Autodesk Inventor part; units mm, degrees
ref_plane "YZ Plane" through (0, 0, 0) normal (1, 0, 0) x (0, 1, 0)
ref_plane "XZ Plane" through (0, 0, 0) normal (0, 1, 0) x (-1, 0, 0)
ref_plane "XY Plane" through (0, 0, 0) normal (0, 0, 1) x (1, 0, 0)
sketch "スケッチ1" plane through (0, 0, 0) normal (0, 0, 1) x (1, 0, 0)
  line L0 (-24.25, -20) -> (24.25, -20) construction
  line L1 (24.25, 20) -> (-24.25, 20)
  line L2 (-24.25, 20) -> (-24.25, -20)
  line L3 (-24.25, -20) -> (24.25, 20) construction
  line L4 (24.25, -20) -> (-24.25, 20) construction
  circle A0 centre (-15.25, -17.5) radius 1.55
  circle A1 centre (20.25, -17.5) radius 1.55
  line L5 (-9.25, -15) -> (14.25, -15) construction
  line L6 (14.25, -15) -> (14.25, -20) construction
  line L7 (14.25, -20) -> (-9.25, -20) construction
  line L8 (-9.25, -20) -> (-9.25, -15) construction
  line L9 (-24.25, -20) -> (-15.25, -22)
  line L10 (-15.25, -22) -> (20.25, -22)
  line L11 (20.25, -22) -> (24.25, -20)
  line L12 (14.3, -14.95) -> (-9.3, -14.95)
  line L13 (-9.3, -14.95) -> (-9.3, -20.05)
  line L14 (-9.3, -20.05) -> (14.3, -20.05)
  line L15 (14.3, -20.05) -> (14.3, -14.95)
  circle A2 centre (-8.25, -14.95) radius 1.05
  circle A3 centre (-8.25, -20.05) radius 1.05
  circle A4 centre (13.25, -14.95) radius 1.05
  circle A5 centre (13.25, -20.05) radius 1.05
  circle A6 centre (-19.25, 15) radius 1.55
  line L16 (-21.8, 5.05) -> (-19.2, 5.05)
  line L17 (-19.2, 5.05) -> (-19.2, -15.05)
  line L18 (-19.2, -15.05) -> (-21.8, -15.05)
  line L19 (-21.8, -15.05) -> (-21.8, 5.05)
  line L20 (-19.25, 5) -> (-21.75, 5) construction
  line L21 (-21.75, 5) -> (-21.75, -15) construction
  line L22 (-21.75, -15) -> (-19.25, -15) construction
  line L23 (-19.25, -15) -> (-19.25, 5) construction
  line L24 (2.5, -14.95) -> (2.5, -20.05) construction
  circle A7 centre (-21.8, 4) radius 1.05
  circle A8 centre (-19.2, 4) radius 1.05
  circle A9 centre (-21.8, -14) radius 1.05
  circle A10 centre (-19.2, -14) radius 1.05
  line L25 (24.25, 9.25) -> (31.25, 9.25)
  line L26 (31.25, 9.25) -> (31.25, -9.25)
  line L27 (31.25, -9.25) -> (24.25, -9.25)
  circle A11 centre (26.25, 0) radius 3.25
  line L28 (24.25, -20) -> (24.25, -9.25)
  line L29 (24.25, 9.25) -> (24.25, 20)
  point P0 (0, 0)
  point P1 (-9.25, -17.5)
  point P2 (12.2, -20.05)
  point P3 (-7.2, -20.05)
  point P4 (-7.2, -14.95)
  point P5 (12.2, -14.95)
  point P6 (-21.8, -12.95)
  point P7 (-21.8, 2.95)
  point P8 (-19.2, 2.95)
  point P9 (-19.2, -12.95)
  dimension "d10" = 2.1
  dimension "d26" = 2.1
  dimension "d0" = 5
  dimension "d3" = 3.1
  dimension "d4" = 35.5
  dimension "d5" = 2
  dimension "d7" = 40
  dimension "d8" = 23.5
  dimension "d9" = 0.05
  dimension "d11" = 3.1
  dimension "d12" = 5
  dimension "d13" = 5
  dimension "d14" = 0.05
  dimension "d15" = 17.75
  dimension "d16" = 48.5
  dimension "d20" = 2.5
  dimension "d21" = 2.5
  dimension "d22" = 5
  dimension "d23" = 15
  dimension "d27" = 25
  dimension "d58" = 6.5
  dimension "d60" = 9.25
  dimension "d61" = 18.5
  dimension "d62" = 20
  dimension "d65" = 2
  dimension "d66" = 5
extrude "押し出し1" add sketch "スケッチ1" along normal blind 5
sketch "スケッチ2" plane through (0, 0, 0) normal (0, 0, -1) x (-1, 0, 0)
  line L0 (-14.3, -20.05) -> (-14.3, -14.95)
  line L1 (-12.2, -14.95) -> (7.2, -14.95)
  line L2 (-24.25, 20) -> (24.25, 20)
  line L3 (-24.25, -20) -> (-24.25, 20)
  line L4 (21.8, -15.05) -> (19.2, -15.05)
  line L5 (19.2, -12.95) -> (19.2, 2.95)
  line L6 (19.2, 5.05) -> (21.8, 5.05)
  line L7 (-20.25, 16) -> (16.25, 16)
  line L8 (16.25, 16) -> (16.25, -11)
  line L9 (16.25, -11) -> (-20.25, -11)
  line L10 (-20.25, -11) -> (-20.25, -5.9161)
  line L11 (-20.25, 16) -> (-20.25, 5.9161)
  line L12 (19.25, 5.05) -> (19.25, -15.05) construction
  line L13 (19.2, -15.05) -> (21.8, -15.05)
  line L14 (-14.3, -15) -> (9.3, -15) construction
  line L15 (9.3, -20.05) -> (9.3, -14.95)
  line L16 (-20.25, 5.9161) -> (-20.25, -5.9161)
  point P0 (0, 0)
  dimension "d29" = 4
  dimension "d30" = 4
  dimension "d31" = 0.05
  dimension "d32" = 3
  dimension "d33" = 0.05
  dimension "d34" = 4
sketch "スケッチ3" plane through (0, 0, 0) normal (0, 0, -1) x (-1, 0, 0)
  circle A0 centre (15.25, -17.5) radius 1.55
  circle A1 centre (15.25, -17.5) radius 3
  circle A2 centre (19.25, 15) radius 1.55
  circle A3 centre (19.25, 15) radius 3
  circle A4 centre (-20.25, -17.5) radius 3
  point P0 (0, 0)
  dimension "d38" = 6
  dimension "d39" = 6
  dimension "d40" = 6
extrude "押し出し3" cut sketch "スケッチ3" against normal blind 3.5 contours A1 | A4
extrude "押し出し5" cut sketch "スケッチ2" against normal blind 3
fillet "フィレット4" radius 2 4 edges at (20.25, -11, 1.5) (20.25, 16, 1.5) (-16.25, 16, 1.5) (-16.25, -11, 1.5)
fillet "フィレット5" radius 2 3 edges at (24.25, -9.25, 2.5) (31.25, -9.25, 2.5) (31.25, 9.25, 2.5)
equation "\"d13\" = d12"
equation "\"d15\" = 0.5 * d4"
equation "\"d60\" = 0.5 * d61"
properties part number "コックピット_サブフレーム_1_5_New" material "アセタール樹脂、黒"
Build history of the part. All positions in model axes, mm. A direction names the side the tool comes from. Give positions to 0.01 mm unless a question says otherwise; leave off trailing zeros. Order: outer loops, then holes, each group sorted by start corner. A loop starts at its lowest first (then second) coordinate and runs counter-clockwise, first axis right, second up. Notation, with made-up numbers: M -33.75,82.25 L 14.25,82.25 A17 cw 14.25,110.25 Z; hole C 13.25,68 d7. An arc over 180 degrees is marked long. Write item = value, one per line. Start each with the question number.
(1) Slice it at B-B on x = -5. Write the cut outline in (y, z).
(2) Slice it at C-C on z = 4.1. State how many separate pieces and enclosed holes the cut face has, plus the area to 3 significant figures.
(3) Pin check, flat tips, straight feed: pin 1 Ø5.5 at (x, y) = (20.25, -17.5) entering from -Z; pin 2 Ø13.5 at (x, y) = (7, -0.5) entering from -Z; pin 3 Ø1.5 at (x, z) = (28.5, 2.5) entering from -Y; pin 4 Ø5 at (x, y) = (26.25, 0) entering from -Z. Stop position of each tip, or through.
(4) Slice it at D-D on y = -17.5. Write the cut outline in (x, z).
(5) Two-plate mould, pull along Y, no slides. Class faces 4 (the flat face through (-24.25, 0, 2)), 5 (the cylindrical face through (24.85, -9.82, 2.54)), 6 (the flat face through (2, -20.05, 2)): released by +Y, released by -Y, zero draft, split by the parting line, or undercut.
(6) Probe L1, parallel to Y at x = -3, z = 0.95; L2, parallel to X at y = 1.5, z = 3.65; L3, parallel to Y at x = -12, z = 1.5. List the from-to ranges inside material, lowest first. Write a range as [from, to].
(7) Which spindle directions (+Z, -Z, +X, -X, +Y, -Y) get a long thin tool onto all of the face, cutting with end or side? Do faces 1 (the cylindrical face through (-15.65, 15.43, 1.52)), 2 (the flat face through (28, -9.25, 2)), 3 (the flat face through (-21, 5.05, 2)). Say none if no direction does.
(8) Slice it at A-A on y = -12. Write the cut outline in (x, z).
Responses:
q1.outline = M -22,0 L -20.05,0 L -20.05,5 L -22,5 Z; M -14.95,0 L -11,0 L -11,3 L 16,3 L 16,0 L 20,0 L 20,5 L -14.95,5 Z
q2.separate_pieces = 1
q2.enclosed_holes = 6
q2.area = 1,910 mm2
q3.pin_1 = 3.5
q3.pin_2 = 3
q3.pin_3 = -9.25
q3.pin_4 = through
q4.outline = M -24.25,0 L -18.25,0 L -18.25,3.5 L -16.8,3.5 L -16.8,5 L -24.25,5 Z; M -13.7,3.5 L -12.25,3.5 L -12.25,0 L -9.3,0 L -9.3,5 L -13.7,5 Z; M 14.3,0 L 17.25,0 L 17.25,3.5 L 18.7,3.5 L 18.7,5 L 14.3,5 Z; M 21.8,3.5 L 23.25,3.5 L 23.25,0 L 24.25,0 L 24.25,5 L 21.8,5 Z
q5.face_4 = zero draft
q5.face_5 = released by -Y
q5.face_6 = undercut
q6.L1 = [-22, -20.05], [-14.95, -11], [16, 20]
q6.L2 = [-24.25, -21.8], [-19.2, 23.37], [29.13, 31.25]
q6.L3 = [-22, -11], [16, 20]
q7.face_1 = -Z
q7.face_2 = +Z, -Z, +X, -Y
q7.face_3 = +Z, -Z
q8.outline = M -24.25,0 L -21.8,0 L -21.8,5 L -24.25,5 Z; M -19.2,0 L 24.25,0 L 24.25,5 L -19.2,5 Z
